Check sheet for the modelled part. Datum: model origin and axes. Units: mm. Coordinates: 2 decimals unless noted, no trailing zeros. Order: outer loops, then holes, each group sorted by start corner. A loop starts at its lowest first (then second) coordinate and runs counter-clockwise, first axis right, second up.
from build123d import *

# Parameters (mm, degrees)
SKETCH1_W           = 25
SKETCH1_H           = 10
BOSS_EXTRUDE1_DEPTH = 10
SKETCH2_R           = 1.6
CUT_EXTRUDE1_DEPTH  = 17.770509831
SKETCH3_R           = 6
CUT_EXTRUDE2_DEPTH  = 25


with BuildPart() as part:
    # Sketch1 → Boss-Extrude1 (new body)
    with BuildSketch(Plane(origin=(0, 0, 0), x_dir=(1, 0, 0), z_dir=(0, 1, 0))):
        Rectangle(SKETCH1_W, SKETCH1_H)
    extrude(amount=BOSS_EXTRUDE1_DEPTH)

    # Sketch2 → Cut-Extrude1 (cut, through all)
    with BuildSketch(Plane(origin=(0, 10, 0), x_dir=(1, 0, 0), z_dir=(0, 1, 0))):
        with Locations(Location((-9.25, 0, 0), (0, 0, 270))):
            Circle(SKETCH2_R)
        with Locations(Location((9.25, 0, 0), (0, 0, 270))):
            Circle(SKETCH2_R)
    extrude(amount=-CUT_EXTRUDE1_DEPTH, mode=Mode.SUBTRACT)

    # Sketch3 → Cut-Extrude2 (cut)
    with BuildSketch(Plane.XY.offset(5)):
        Circle(SKETCH3_R)
    extrude(amount=-CUT_EXTRUDE2_DEPTH, mode=Mode.SUBTRACT)


solid = part.part
(1) Cross-section at B-B (x = 9.25). Enter the section's corners in (y, z), and give its area (3 significant figures).
Filled in:
outline: (0, -5) - (10, -5) - (10, -1.6) - (0, -1.6) - close; (0, 1.6) - (10, 1.6) - (10, 5) - (0, 5) - close
area: 68.0 mm2
(2) Cross-section at A-A (z = 0). Enter the section's corners in (x, y), and give its area (3 significant figures).
Filled in:
outline: (-12.5, 0) - (-10.85, 0) - (-10.85, 10) - (-12.5, 10) - close; (-7.65, 0) - (-6, 0) arc R6 cw to (6, 0) - (7.65, 0) - (7.65, 10) - (-7.65, 10) - close; (10.85, 0) - (12.5, 0) - (12.5, 10) - (10.85, 10) - close
area: 129 mm2
(3) Cross-section at C-C (y = 8.5). Enter the section's corners in (x, z).
Filled in:
outline: (-12.5, -5) - (12.5, -5) - (12.5, 5) - (-12.5, 5) - close; hole circle Ø3.2 at (-9.25, 0); hole circle Ø3.2 at (9.25, 0)
(4) Thickness scan on probe 1 along X at (y, z) = (5, 0); probe 2 along X at (y, z) = (3.25, -0.5); probe 3 along X at (y, z) = (1.5, -3). Record the ranges inside material, lowest first.
Filled in:
probe 1: x = -12.5 to -10.85, -7.65 to -3.32, 3.32 to 7.65, 10.85 to 12.5
probe 2: x = -12.5 to -10.77, -7.73 to -5.04, 5.04 to 7.73, 10.77 to 12.5
probe 3: x = -12.5 to -5.81, 5.81 to 12.5
(5) Cross-section at D-D (y = 1.25). Enter the section's corners in (x, z).
Filled in:
outline: (-12.5, -5) - (-5.87, -5) - (-5.87, 5) - (-12.5, 5) - close; (5.87, -5) - (12.5, -5) - (12.5, 5) - (5.87, 5) - close; hole circle Ø3.2 at (-9.25, 0); hole circle Ø3.2 at (9.25, 0)
(6) Release check for a two-part mould opening along X. For faces 1 (the cylindrical face through (7.69, 5.07, -0.35)), 2 (the cylindrical face through (0, 6, 0)), 3 (the flat face through (-11, 0, 1)), 4 (the flat face through (-12.5, 5, 0)) record: +X half, -X half, draft (parallel to the pull), parting line (faces both ways), or undercut.
Filled in:
face 1: undercut
face 2: undercut
face 3: draft
face 4: -X half
